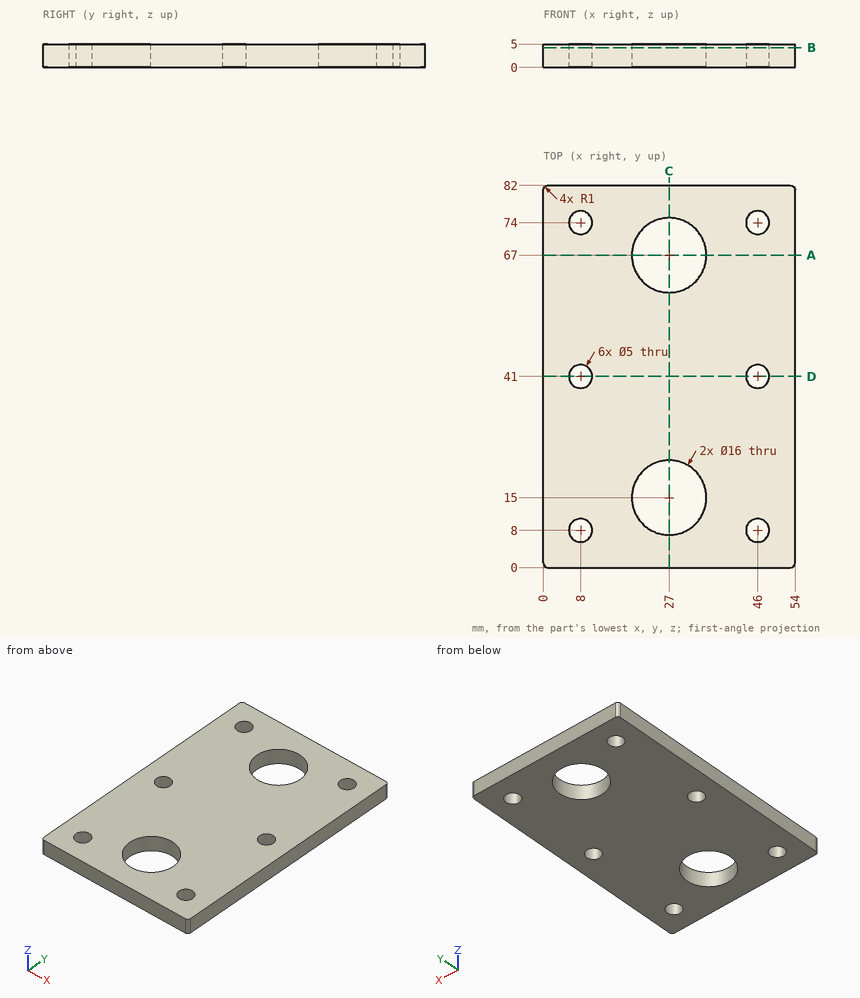
Here's the drawing with two shaded views (mm, measured from the low corner). I have some questions. Coordinates: 2 decimals unless noted, no trailing zeros. Write each loop counter-clockwise with the first axis right and the second up, starting at its lowest first coordinate (ties: lowest second). Pieces come first, ordered by that corner, then holes. Notation, with made-up numbers: (-17.75, 22) -> (20.25, 22) arc R15 ccw to (20.25, 30) -> close; hole circle Ø1 at (61.25, 65.25). An arc over 180 degrees is marked (long way). Use a Markdown table: item, result. Add a question column.
(1) If we section it at B-B, the plane z = 4.2: State how many separate pieces and enclosed holes the cut face has, and give its area (3 significant figures).
(2) Please list where these lines run through material, in increasing order: line 1 (Y direction, x = 46, z = 3.8); line 2 (X direction, y = 9, z = 4.8); line 3 (X direction, y = 6.5, z = 0.8).
(3) If we section it at D-D, the plane y = 41: Write out the boundary of the cut face in (x, z), and give its area (3 significant figures).
(4) If we section it at C-C, the plane x = 27: Write out the boundary of the cut face in (y, z).
(5) If we section it at A-A, the plane y = 67: Write out the boundary of the cut face in (x, z).
(6) I'm going to push a flat-ended pin straight in: P1, Ø6.5, axis at x = 46, y = 74, coming from the -Z side. Where does the tip first touch, or does it pass through?
Outcome:
| question | item | result |
|---|---|---|
| 1 | separate pieces | 1 |
| 1 | enclosed holes | 8 |
| 1 | area | 3,910 mm^2 |
| 2 | line 1 | y = 0 to 5.5, 10.5 to 38.5, 43.5 to 71.5, 76.5 to 82 |
| 2 | line 2 | x = 0 to 5.71, 10.29 to 21.71, 32.29 to 43.71, 48.29 to 54 |
| 2 | line 3 | x = 0 to 6, 10 to 44, 48 to 54 |
| 3 | outline | (0, 0) -> (5.5, 0) -> (5.5, 5) -> (0, 5) -> close; (10.5, 0) -> (43.5, 0) -> (43.5, 5) -> (10.5, 5) -> close; (48.5, 0) -> (54, 0) -> (54, 5) -> (48.5, 5) -> close |
| 3 | area | 220 mm^2 |
| 4 | outline | (0, 0) -> (7, 0) -> (7, 5) -> (0, 5) -> close; (23, 0) -> (59, 0) -> (59, 5) -> (23, 5) -> close; (75, 0) -> (82, 0) -> (82, 5) -> (75, 5) -> close |
| 5 | outline | (0, 0) -> (19, 0) -> (19, 5) -> (0, 5) -> close; (35, 0) -> (54, 0) -> (54, 5) -> (35, 5) -> close |
| 6 | P1 | stops at z = 0 |
